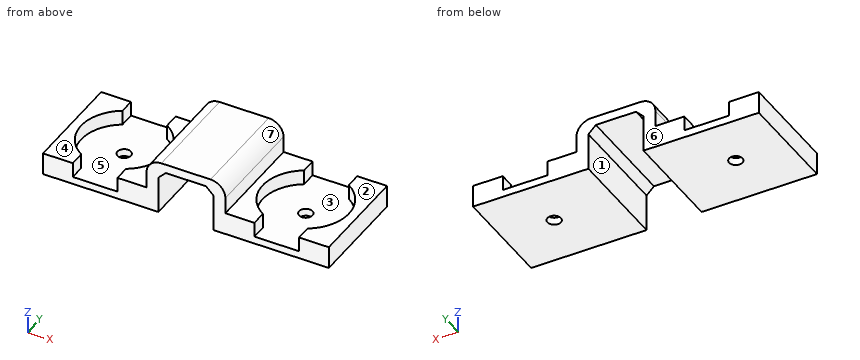
from build123d import *

# Parameters (mm, degrees)
PAD_DEPTH       = 7
SKETCH006_W     = 14
SKETCH006_H     = 14
PAD002_DEPTH    = 3
POCKET004_DEPTH = 2
SKETCH008_R     = 0.9
POCKET005_DEPTH = 1.001
FILLET001_R     = 2
CHAMFER_SIZE    = 1


with BuildPart() as clamp_unit001:
    # Sketch → Pad (new body, symmetric)
    with BuildSketch(Plane.XZ):
        Polygon((-3.7, 7.2), (5.3, 7.2), (5.3, 0), (3.7, 0), (3.7, 6), (-3.7, 6), (-3.7, 0), (-5.3, 0), (-5.3, 7.2), align=None)
    extrude(amount=PAD_DEPTH, both=True)


with BuildPart() as obj1:
    # Sketch006 → Pad002 (new body)
    with BuildSketch(Plane.XY):
        Rectangle(SKETCH006_W, SKETCH006_H)
    extrude(amount=PAD002_DEPTH)

    # Sketch007 (on Face6 of Pad002) → Pocket004 (cut)
    with BuildSketch(Plane.XY.offset(3)):
        with BuildLine():
            Line((-3, 7), (-3, 4.963869))
            ThreePointArc((-3, 4.963869), (-5.8, 0), (-3, -4.963869))
            Line((-3, -7), (-3, -4.963869))
            Line((3, -7), (-3, -7))
            Line((3, -4.963869), (3, -7))
            ThreePointArc((3, -4.963869), (5.8, 0), (3, 4.963869))
            Line((3, 7), (3, 4.963869))
            Line((-3, 7), (3, 7))
        make_face()
    extrude(amount=-POCKET004_DEPTH, mode=Mode.SUBTRACT)

    # Sketch008 (on Face6 of Pocket004) → Pocket005 (cut, through all)
    with BuildSketch(Plane.XY.offset(1)):
        Circle(SKETCH008_R)
    extrude(amount=-POCKET005_DEPTH, mode=Mode.SUBTRACT)


with BuildPart() as obj1_1:
    # Clone placement: moved
    add(obj1.part.moved(Location((-11.2, 0, 0))))


with BuildPart() as obj1_2:
    # Clone002 placement: moved
    add(obj1_1.part.moved(Location((-1, 0, 0))))


with BuildPart() as obj2:
    # Clone004 base: copy of obj1
    add(obj1_2.part)


with BuildPart() as obj2_1:
    # Clone004 placement: moved
    add(obj2.part.moved(Location((24.4, 0, 0))))


with BuildPart() as obj3:
    # Fusion001 base: copy of obj1
    add(obj1_2.part)

    # Fusion001: union clamp-unit001, obj2
    add(clamp_unit001.part)
    add(obj2_1.part)

    # Fillet001
    fillet001_edges = [obj3.edges().sort_by_distance(p)[0] for p in [
        (5.3, 0, 7.2),
        (-5.3, 0, 7.2),
    ]]
    fillet(fillet001_edges, radius=FILLET001_R)

    # Chamfer
    chamfer_edges = [obj3.edges().sort_by_distance(p)[0] for p in [
        (-3.7, 0, 6),
        (3.7, 0, 6),
    ]]
    chamfer(chamfer_edges, length=CHAMFER_SIZE)


solid = obj3.part
Work out the finished part from the listing and answer in its coordinate system (mm). Face numbers are marked on the shaded views. A direction names the side the tool comes from. Round coordinates to 2 decimals unless told otherwise and drop trailing zeros. Write each loop counter-clockwise with the first axis right and the second up, starting at its lowest first coordinate (ties: lowest second). Pieces come first, ordered by that corner, then holes.
1) A cutting plane is placed at B-B (z = 4). Give the vertices of the cut face in (x, y).
2) The mould has two halves that part along X. Classify the marked faces 5, 6 and 7: pulls with the +X half, pulls with the -X half, needs draft (parallel to the pull), parting line crosses it, or undercut.
3) A cutting plane is placed at C-C (y = 0). Give the number of separate pieces and of enclosed holes in the cut face, plus the area to 3 significant figures.
4) A cutting plane is placed at D-D (z = 2.5). Give the vertices of the cut face in (x, y), plus the area to 3 significant figures.
5) A tool of negligible diameter and unlimited length cuts with its end or side. For the marked faces 1, 2, 3 and 4, from which of +Z, -Z, +X, -X, +Y, -Y can it reach the whole face along a straight path? Write none if from no direction.
6) A cutting plane is placed at A-A (x = -12.2). Give the vertices of the cut face in (y, z).
7) Straight lines are drawn through the part: line 1 (Y direction, x = 12.2, z = 0.45); line 2 (X direction, y = -5.25, z = 1.75); line 3 (X direction, y = 4, z = 4). For each, find the intervals that lie inside material, in ascending order.
8) Given pin 1 Ø2.5 at (y, z) = (-3, 4) entering from -X; pin 2 Ø3 at (x, y) = (-12.2, 0) entering from +Z; pin 3 Ø2 at (x, y) = (-18, 1) entering from +Z; pin 4 Ø0.7 at (y, z) = (2, 3.5) entering from +X, each flat-ended and moving along its own axis, determine where each tip first touches the part or whether it passes through.
Completed:
1. outline: (-5.3, -7) - (-3.7, -7) - (-3.7, 7) - (-5.3, 7) - close; (3.7, -7) - (5.3, -7) - (5.3, 7) - (3.7, 7) - close
2. face 5: undercut
2. face 6: needs draft
2. face 7: pulls with the +X half
3. separate pieces: 3
3. enclosed holes: 0
3. area: 64.6 mm2
4. outline: (-19.2, -7) - (-15.2, -7) - (-15.2, -4.96) arc R5.8 cw to (-15.2, 4.96) - (-15.2, 7) - (-19.2, 7) - close; (-9.2, -7) - (-3.7, -7) - (-3.7, 7) - (-9.2, 7) - (-9.2, 4.96) arc R5.8 cw to (-9.2, -4.96) - close; (3.7, -7) - (9.2, -7) - (9.2, -4.96) arc R5.8 cw to (9.2, 4.96) - (9.2, 7) - (3.7, 7) - close; (15.2, -7) - (19.2, -7) - (19.2, 7) - (15.2, 7) - (15.2, 4.96) arc R5.8 cw to (15.2, -4.96) - close
4. area: 187 mm2
5. face 1: -Z, +Y, -Y
5. face 2: +Z, +X, +Y, -Y
5. face 3: +Z
5. face 4: +Z, -X, +Y, -Y
6. outline: (-7, 0) - (-0.9, 0) - (-0.9, 1) - (-7, 1) - close; (0.9, 0) - (7, 0) - (7, 1) - (0.9, 1) - close
7. line 1: y = -7 to -0.9, 0.9 to 7
7. line 2: x = -19.2 to -15.2, -9.2 to -3.7, 3.7 to 9.2, 15.2 to 19.2
7. line 3: x = -5.3 to -3.7, 3.7 to 5.3
8. pin 1: stops at x = -19.2
8. pin 2: stops at z = 1
8. pin 3: stops at z = 3
8. pin 4: stops at x = 5.3
